The listing builds one solid part. Answer for the finished solid, in the listing's coordinates (mm). Face numbers are marked on the shaded views. A direction names the side the tool comes from. Round coordinates to 2 decimals unless told otherwise and drop trailing zeros. Order: outer loops, then holes, each group sorted by start corner. A loop starts at its lowest first (then second) coordinate and runs counter-clockwise, first axis right, second up. Notation, with made-up numbers: (-8.75, -35) -> (18.25, -35) arc R18 ccw to (18.25, -29) -> close; hole circle Ø7 at (72.5, -1.5). An arc over 180 degrees is marked (long way). Answer in a Markdown table with one row per item. Add a question column.
```python
from build123d import *

# Parameters (mm, degrees)
F0_R     = 10.795
F0_R_2   = 9.1821
F0_R_3   = 4.826
F1_DEPTH = 60.96
F2_DEPTH = 69.342
F3_DEPTH = 60.96
F4_DEPTH = 69.342


with BuildPart() as f1:
    # F0 (on Front) → F1 (new body)
    with BuildSketch(Plane.XZ):
        Circle(F0_R)
        Circle(F0_R_2, mode=Mode.SUBTRACT)
        Circle(F0_R_2)
        Circle(F0_R_3, mode=Mode.SUBTRACT)
        Circle(F0_R_3)
    extrude(amount=F1_DEPTH)

    # F0 (on Front) → F2 (join)
    with BuildSketch(Plane.XZ):
        Circle(F0_R_3)
    extrude(amount=F2_DEPTH)

    # F0 (on Front) → F3 (join)
    with BuildSketch(Plane.XZ):
        Circle(F0_R_2)
        Circle(F0_R_3, mode=Mode.SUBTRACT)
        Circle(F0_R_3)
    extrude(amount=-F3_DEPTH)

    # F0 (on Front) → F4 (join)
    with BuildSketch(Plane.XZ):
        Circle(F0_R_3)
    extrude(amount=-F4_DEPTH)


solid = f1.part
```
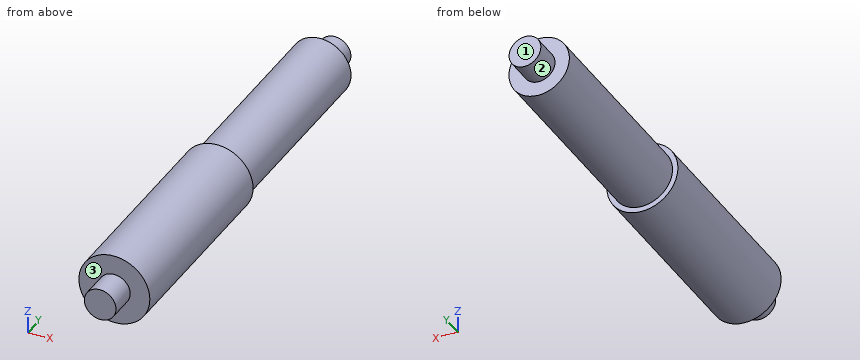
1. For the marked faces 1, 2 and 3, determine the directions among +Z, -Z, +X, -X, +Y, -Y from which every point of the face is accessible in a straight line to the end or side of a thin tool.
2. The part is cut by section C-C (y = 39). Give the vertices of the cut face in (x, z), then the cut area to 3 significant figures.
3. The part is cut by section B-B (x = 0). Give the vertices of the cut face in (y, z) (3 decimals), then the cut area to 3 significant figures.
4. The part is cut by section A-A (z = 0). Give the vertices of the cut face in (x, y) (3 decimals).
5. The part is cut by section D-D (x = -7.5). Give the vertices of the cut face in (y, z).
6. Straight lines are drawn through the part: line 1 along Y through (x, z) = (3.5, -10); line 2 along X through (y, z) = (-53.5, -0.25); line 3 along Y through (x, z) = (-0.25, 8.75). For each, find the intervals that lie inside material, in ascending order.
7. Each of these flat-tipped pins is pushed along its axis until it touches: pin 1 (5 mm diameter, centred on y = -19.5, z = -5, fed in from +X); pin 2 (2 mm diameter, centred on x = -7.5, z = -8, fed in from +Y); pin 3 (2 mm diameter, centred on x = -3, y = -18.5, fed in from -Z). Where does it stop, or does it pass through?
Report:
| question | item | result |
|---|---|---|
| 1 | face 1 | +Z, -Z, +X, -X, +Y |
| 1 | face 2 | +Y |
| 1 | face 3 | -Y |
| 2 | outline | circle Ø18.36 at (0, 0) |
| 2 | area | 265 mm^2 |
| 3 | outline | (-69.342, -4.826) -> (-60.96, -4.826) -> (-60.96, -10.795) -> (0, -10.795) -> (0, -9.182) -> (60.96, -9.182) -> (60.96, -4.826) -> (69.342, -4.826) -> (69.342, 4.826) -> (60.96, 4.826) -> (60.96, 9.182) -> (0, 9.182) -> (0, 10.795) -> (-60.96, 10.795) -> (-60.96, 4.826) -> (-69.342, 4.826) -> close |
| 3 | area | 2,600 mm^2 |
| 4 | outline | (-10.795, -60.96) -> (-4.826, -60.96) -> (-4.826, -69.342) -> (4.826, -69.342) -> (4.826, -60.96) -> (10.795, -60.96) -> (10.795, 0) -> (9.182, 0) -> (9.182, 60.96) -> (4.826, 60.96) -> (4.826, 69.342) -> (-4.826, 69.342) -> (-4.826, 60.96) -> (-9.182, 60.96) -> (-9.182, 0) -> (-10.795, 0) -> close |
| 5 | outline | (-60.96, -7.76) -> (0, -7.76) -> (0, -5.3) -> (60.96, -5.3) -> (60.96, 5.3) -> (0, 5.3) -> (0, 7.76) -> (-60.96, 7.76) -> close |
| 6 | line 1 | y = -60.96 to 0 |
| 6 | line 2 | x = -10.79 to 10.79 |
| 6 | line 3 | y = -60.96 to 60.96 |
| 7 | pin 1 | stops at x = 10.5 |
| 7 | pin 2 | stops at y = 0 |
| 7 | pin 3 | stops at z = -10.61 |
